Design review of the part built by this model. Coordinates are the model's own, in mm. Give positions to 0.01 mm unless a question says otherwise; leave off trailing zeros. Loops run counter-clockwise (first coordinate to the right, second up) from the corner with the lowest first, then second, coordinate; pieces in that order, holes last. Notation, with made-up numbers: (9.5, 89.25) -> (28.5, 89.25) arc R13 cw to (28.5, 93.25) -> close; hole circle Ø8 at (12, 87). An arc over 180 degrees is marked (long way). Answer in a Markdown table with one row per item. Add a question column.
(1) Consider section C-C on x = 5.5. Write out the cut boundary in (y, z), then the cut area to 3 significant figures.
(2) For pin 1 (5 mm diameter, centred on y = -107, z = -1, fed in from -X); pin 2 (1.5 mm diameter, centred on y = -79, z = 0.5, fed in from +X), all flat-tipped, find the tip position at first contact; note any pin that passes through.
(3) Consider section A-A on z = -3. Write out the cut boundary in (x, y).
(4) For line 1 (Y direction, x = 81, z = -0.75); line 2 (Y direction, x = 98.5, z = -2.5); line 3 (X direction, y = -117.5, z = -2), list the stretches that pass through material, from the lowest coordinate up.
(5) Consider section B-B on y = -132. Write out the cut boundary in (x, z), then the cut area to 3 significant figures.
from build123d import *

# Parameters (mm, degrees)
BOSS_EXTRUDE1_DEPTH = 5
FILLET1_R           = 5


with BuildPart() as part:
    # Sketch1 → Boss-Extrude1 (new, symmetric)
    with BuildSketch(Plane.XY):
        Polygon((-12.672945593, -60.23903484), (148.589587107, -60.23903484), (53.589587107, -155.23903484), (7.97922832, -155.23903484), align=None)
    extrude(amount=BOSS_EXTRUDE1_DEPTH, both=True)

    # Fillet1
    fillet1_edges = [part.edges().sort_by_distance(p)[0] for p in [
        (-12.672945593, -60.23903484, 0),
        (148.589587107, -60.23903484, 0),
        (53.589587107, -155.23903484, 0),
        (7.97922832, -155.23903484, 0),
    ]]
    fillet(fillet1_edges, radius=FILLET1_R)


solid = part.part
Values follow:
| question | item | result |
|---|---|---|
| 1 | outline | (-143.83, -5) -> (-60.24, -5) -> (-60.24, 5) -> (-143.83, 5) -> close |
| 1 | area | 836 mm2 |
| 2 | pin 1 | x = -3.05 |
| 2 | pin 2 | x = 130.58 |
| 3 | outline | (-11.36, -66.3) -> (7.12, -151.3) arc R5 ccw to (12.01, -155.24) -> (51.52, -155.24) arc R5 ccw to (55.05, -153.77) -> (140.05, -68.77) arc R5 ccw to (136.52, -60.24) -> (-6.47, -60.24) arc R5 ccw to start |
| 4 | line 1 | -127.83 to -60.24 |
| 4 | line 2 | -110.33 to -60.24 |
| 4 | line 3 | -0.22 to 91.33 |
| 5 | outline | (2.93, -5) -> (76.83, -5) -> (76.83, 5) -> (2.93, 5) -> close |
| 5 | area | 739 mm2 |
